```python
from build123d import *

# Parameters (mm, degrees)
SKETCH1_W             = 101.1682
SKETCH1_H             = 6.35
SKETCH1_W_2           = 6.35
SKETCH1_H_2           = 170.072742275
BOSS_EXTRUDE1_DEPTH   = 6.35
F_8_CLEARANCE_HOLE1_D = 4.4958


with BuildPart() as part:
    # Sketch1 → Boss-Extrude1 (new body)
    with BuildSketch(Plane.XY):
        with BuildLine():
            Line((25.4, -12.7), (-139.2682, -12.7))
            ThreePointArc((-139.2682, -12.7), (-143.758328061, -10.840128061), (-145.6182, -6.35))
            Line((-145.6182, -6.35), (-145.6182, 201.822742275))
            ThreePointArc((-145.6182, 201.822742275), (-143.758328061, 206.312870335), (-139.2682, 208.172742275))
            Line((-139.2682, 208.172742275), (25.4, 208.172742275))
            ThreePointArc((25.4, 208.172742275), (29.890128061, 206.312870335), (31.75, 201.822742275))
            Line((31.75, 201.822742275), (31.75, -6.35))
            ThreePointArc((31.75, -6.35), (29.890128061, -10.840128061), (25.4, -12.7))
        make_face()
        with Locations((-56.9341, 192.297742275)):
            Rectangle(SKETCH1_W, SKETCH1_H, mode=Mode.SUBTRACT)
        with Locations((3.175, 97.736371138)):
            Rectangle(SKETCH1_W_2, SKETCH1_H_2, mode=Mode.SUBTRACT)
        with Locations((-117.0432, 97.736371138)):
            Rectangle(SKETCH1_W_2, SKETCH1_H_2, mode=Mode.SUBTRACT)
        with Locations((-56.9341, 104.775)):
            Rectangle(SKETCH1_W, SKETCH1_H, mode=Mode.SUBTRACT)
        with Locations((-56.9341, 3.175)):
            Rectangle(SKETCH1_W, SKETCH1_H, mode=Mode.SUBTRACT)
        with Locations((-56.9341, 51.6128)):
            Rectangle(SKETCH1_W, SKETCH1_H, mode=Mode.SUBTRACT)
    extrude(amount=BOSS_EXTRUDE1_DEPTH)

    # #8 Clearance Hole1 (through all)
    with Locations(Plane(origin=(-70.641043598, 181.536765785, 9.525), x_dir=(-1, 0, 0), z_dir=(0, 0, 1))):
        with Locations((62.625233431, 162.765803656), (62.772094273, 9.954588756), (-90.039120627, 9.807727914), (-90.185981469, 162.618942814)):
            Hole(F_8_CLEARANCE_HOLE1_D / 2)


solid = part.part
```
The listing builds one solid part. Answer for the finished solid, in the listing's coordinates (mm). A direction names the side the tool comes from. Coordinates: 2 decimals unless noted, no trailing zeros. Write each loop counter-clockwise with the first axis right and the second up, starting at its lowest first coordinate (ties: lowest second). Pieces come first, ordered by that corner, then holes. Notation, with made-up numbers: (36.25, -25.75) - (91.25, -25.75) arc R25 ccw to (91.25, -0.75) - close; hole circle Ø8 at (-14, 46). An arc over 180 degrees is marked (long way). Return JSON: item names as keys, results as strings. Group by question number.
Q1. Which of the six approach directions +Z, -Z, +X, -X, +Y, -Y give full straight-line access (tool end or side, diameter ignored) to faces 1 (the cylindrical face through (-143.81, 206.26, 3.13)), 2 (the flat face through (-6.35, 52, 3))?
Q2. The part is cut by section B-B on y = 90.5. Write down the section's boundary in (x, z), and give its area (3 significant figures).
Q3. The part is cut by section C-C on z = 3. State how many separate pieces and enclosed holes the cut face has, and give its area (3 significant figures).
Q4. A flat-ended cylindrical pin translates along its axis: pin 1 Ø2.5 at (x, y) = (19.54, 18.92) entering from +Z. Find the tip coordinate at first contact, or state that the pin passes through.
Q5. Find the intervals of material crossed by line 1 along X through (y, z) = (43.5, 6); line 2 along Y through (x, z) = (-45, 3); line 3 along Y through (x, z) = (-114, 2.25), in increasing order. Write a range as [from, to].
Q6. The part is cut by section A-A on x = -26.5. Write down the section's boundary in (y, z), and give its area (3 significant figures).
Q7. For a pull along Y with two mould halves and no side action, classify faces 3 (the cylindrical face through (19.058, 21.112, 3.131)), 4 (the flat face through (-107.518, 3, 3)), 5 (the flat face through (-56, 99, 6.35)), 6 (the cylindrical face through (29.8, 206.4, 3.1)) as +Y half, -Y half, draft (parallel to the pull), parting line (faces both ways), or undercut.
Evaluation:
{
 "1": {"face 1": "+Z, -Z, -X, +Y", "face 2": "+Z, -Z"},
 "2": {"outline": "(-145.62, 0) - (-120.22, 0) - (-120.22, 6.35) - (-145.62, 6.35) - close; (-113.87, 0) - (0, 0) - (0, 6.35) - (-113.87, 6.35) - close; (6.35, 0) - (31.75, 0) - (31.75, 6.35) - (6.35, 6.35) - close", "area": "1,050 mm2"},
 "3": {"separate pieces": "1", "enclosed holes": "10", "area": "34,300 mm2"},
 "4": {"pin 1": "passes through"},
 "5": {"line 1": "x = [-145.62, -120.22], [-113.87, 0], [6.35, 31.75]", "line 2": "y = [-12.7, 0], [6.35, 48.44], [54.79, 101.6], [107.95, 189.12], [195.47, 208.17]", "line 3": "y = [-12.7, 12.7], [182.77, 208.17]"},
 "6": {"outline": "(-12.7, 0) - (0, 0) - (0, 6.35) - (-12.7, 6.35) - close; (6.35, 0) - (48.44, 0) - (48.44, 6.35) - (6.35, 6.35) - close; (54.79, 0) - (101.6, 0) - (101.6, 6.35) - (54.79, 6.35) - close; (107.95, 0) - (189.12, 0) - (189.12, 6.35) - (107.95, 6.35) - close; (195.47, 0) - (208.17, 0) - (208.17, 6.35) - (195.47, 6.35) - close", "area": "1,240 mm2"},
 "7": {"face 3": "undercut", "face 4": "undercut", "face 5": "draft", "face 6": "+Y half"}
}
